```python
from build123d import *

# Parameters (mm, degrees)
SKETCH_1_R      = 17.5
SKETCH_1_R_2    = 3
EXTRUDE_1_DEPTH = 10
EXTRUDE_START   = -10
SKETCH_2_R      = 40
SKETCH_2_R_2    = 17.5
EXTRUDE_3_DEPTH = 10


with BuildPart() as part:
    # 草图1 → 凸台-拉伸1 (new body)
    with BuildSketch(Plane.XY):
        Circle(SKETCH_1_R)
        with Locations((-12, 0)):
            Circle(SKETCH_1_R_2, mode=Mode.SUBTRACT)
        with Locations((0, 12)):
            Circle(SKETCH_1_R_2, mode=Mode.SUBTRACT)
        with Locations((12, 0)):
            Circle(SKETCH_1_R_2, mode=Mode.SUBTRACT)
        with Locations((0, -12)):
            Circle(SKETCH_1_R_2, mode=Mode.SUBTRACT)
    extrude(amount=EXTRUDE_1_DEPTH)

    # 草图2 → 凸台-拉伸3 (add)
    with BuildSketch(Plane.XY.offset(10).offset(EXTRUDE_START)):
        Circle(SKETCH_2_R)
        Circle(SKETCH_2_R_2, mode=Mode.SUBTRACT)
    extrude(amount=EXTRUDE_3_DEPTH)


solid = part.part
```
The listing builds one solid part. Answer for the finished solid, in the listing's coordinates (mm). Round coordinates to 2 decimals unless told otherwise and drop trailing zeros. Order: outer loops, then holes, each group sorted by start corner. A loop starts at its lowest first (then second) coordinate and runs counter-clockwise, first axis right, second up. Notation, with made-up numbers: (83, 67.5) - (131, 67.5) arc R32 ccw to (131, 93.5) - close; hole circle Ø9 at (34, 27.5). An arc over 180 degrees is marked (long way). Put each result on its own line as item: value. Start each with the question number.
(1) Given P1, Ø5, axis at x = -12, y = 0, coming from the -Z side; P2, Ø3, axis at y = -18, z = 2.5, coming from the +X side; P3, Ø6, axis at y = 28.5, z = 4, coming from the -X side; P4, Ø3, axis at x = 21, z = 2.5, coming from the -Y side, each flat-ended and moving along its own axis, determine where each tip first touches the part or whether it passes through.
(2) Straight lines are drawn through the part: probe 1 along X at (y, z) = (-2.5, 1.25); probe 2 along Y at (x, z) = (10.5, 8.75); probe 3 along Y at (x, z) = (-14, 7.75). For each, find the intervals that lie inside material, in ascending order. Write a range as from..to.
(3) Determine the mould class of faces 1 (the cylindrical face through (-0.65, -14.93, 4.93)), 2 (the cylindrical face through (-8.67, -39.05, 4.93)), 3 (the flat face through (-1, 1, 10)) for opening direction X: released by +X, released by -X, zero draft, split by the parting line, or undercut.
(4) Find section C-C (x = -12). Give the vertices of the cut face in (y, z), plus the area to 3 significant figures.
(5) Find section B-B (z = 8). Give the vertices of the cut face in (x, y).
(6) Find section A-A (x = 0). Give the vertices of the cut face in (y, z).
Reply:
1. P1: through
1. P2: x = 36.44
1. P3: x = -30.82
1. P4: y = -34.92
2. probe 1: -39.92..-13.66, -10.34..10.34, 13.66..39.92
2. probe 2: -38.6..-2.6, 2.6..38.6
2. probe 3: -37.47..-2.24, 2.24..37.47
3. face 1: undercut
3. face 2: split by the parting line
3. face 3: zero draft
4. outline: (-38.16, 0) - (-3, 0) - (-3, 10) - (-38.16, 10) - close; (3, 0) - (38.16, 0) - (38.16, 10) - (3, 10) - close
4. area: 703 mm^2
5. outline: circle Ø80 at (0, 0); hole circle Ø6 at (-12, 0); hole circle Ø6 at (0, -12); hole circle Ø6 at (0, 12); hole circle Ø6 at (12, 0)
6. outline: (-40, 0) - (-15, 0) - (-15, 10) - (-40, 10) - close; (-9, 0) - (9, 0) - (9, 10) - (-9, 10) - close; (15, 0) - (40, 0) - (40, 10) - (15, 10) - close
